Autodesk Inventor part; units mm, degrees
ref_plane "YZ Plane" through (0, 0, 0) normal (1, 0, 0) x (0, 1, 0)
ref_plane "XZ Plane" through (0, 0, 0) normal (0, 1, 0) x (-1, 0, 0)
ref_plane "XY Plane" through (0, 0, 0) normal (0, 0, 1) x (1, 0, 0)
sketch "Profile" plane through (0, 0, 0) normal (0, 0, 1) x (1, 0, 0)
  line L0 (-22.8, 0) -> (-22.8, 11)
  line L1 (-22.8, 11) -> (0, 11)
  line L2 (0, 11) -> (0.5774, 12)
  line L3 (0.5774, 12) -> (48.0774, 12)
  line L4 (48.0774, 12) -> (48.6547, 11)
  line L5 (48.6547, 11) -> (72.2, 11)
  line L6 (72.2, 11) -> (72.2, 0)
  line L7 (-22.8, 0) -> (0, 0)
  line L8 (0, 0) -> (0, 9)
  line L9 (0, 9) -> (64.2, 9)
  line L10 (64.2, 9) -> (64.2, 0)
  line L11 (64.2, 0) -> (72.2, 0)
  line L12 (-41.8, 0) -> (91.2, 0) construction
  line L13 (0, 11) -> (0, 9) construction
  dimension "BodyLength" = 95
  dimension "d1" = 11
  dimension "d3" = 120
  dimension "d4" = 120
  dimension "d5" = 47.5
  dimension "d6" = 22.8
  dimension "d16" = 8
  dimension "d29" = 1
  dimension "d30" = 9
revolve "ProfileRevolveFeature" add sketch "Profile" angle 360 about axis through (-10, 0, 0) along (1, 0, 0)
sketch "InsideHole" plane through (-22.8, 0, 0) normal (-1, 0, 0) x (0, 0, 1)
  circle A0 centre (0, 0) radius 9 construction
hole "InsideHoleFeature" at (-22.8, 0, 0) direction (1, 0, 0) diameter 19 end through all
chamfer "EndChamferFeature" distance 1 angle 45 1 edges at (-22.8, -11, 0)
sketch "CapMountHole" plane through (0, 0, 0) normal (0, 1, 0) x (-1, 0, 0)
  line L0 (-72.2, 11) -> (-72.2, -11) construction
  line L1 (15.2, 0) -> (-91.2, 0) construction
  circle A0 centre (-67.7, 0) radius 1.25
  point P0 (0, 0)
  dimension "d31" = 4.5
  dimension "d39" = 2.5
extrude "CapMountHoleFeature" cut sketch "CapMountHole" along normal through all both and the other way through all
equation "\"d5\" = 0.5 * BodyLength"
equation "\"d6\" = 0.24 * BodyLength"
properties part number "BackPair1PistonBody"
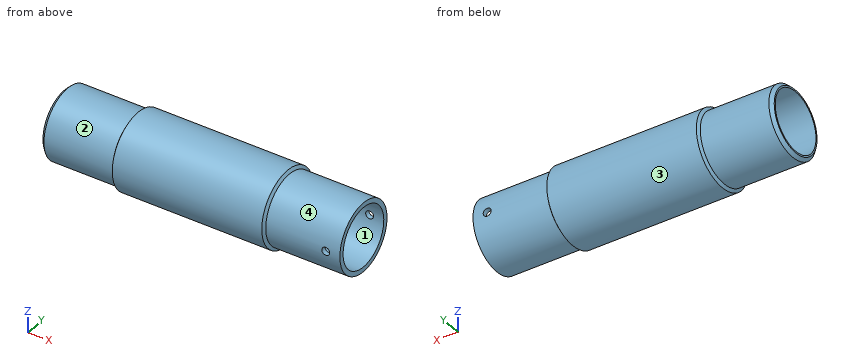
Could you check a few things on this model? Use its own coordinates, in mm. Face numbers are marked on the shaded views. A direction names the side the tool comes from. Round coordinates to 2 decimals unless told otherwise and drop trailing zeros. Order: outer loops, then holes, each group sorted by start corner. A loop starts at its lowest first (then second) coordinate and runs counter-clockwise, first axis right, second up.
(1) Imagine slicing it at B-B (z = 0). Write out the boundary of the cut face in (x, y), plus the area to 3 significant figures.
Response values:
outline: (-22.8, -10) - (-21.8, -11) - (0, -11) - (0.58, -12) - (48.08, -12) - (48.65, -11) - (66.45, -11) - (66.45, -9.5) - (-22.8, -9.5) - close; (-22.8, 9.5) - (66.45, 9.5) - (66.45, 11) - (48.65, 11) - (48.08, 12) - (0.58, 12) - (0, 11) - (-21.8, 11) - (-22.8, 10) - close; (68.95, -11) - (72.2, -11) - (72.2, -9.5) - (68.95, -9.5) - close; (68.95, 9.5) - (72.2, 9.5) - (72.2, 11) - (68.95, 11) - close
area: 373 mm2
(2) Imagine slicing it at A-A (y = 0). Write out the boundary of the cut face in (x, z), plus the area to 3 significant figures.
Response values:
outline: (-22.8, -10) - (-21.8, -11) - (0, -11) - (0.58, -12) - (48.08, -12) - (48.65, -11) - (72.2, -11) - (72.2, -9.5) - (-22.8, -9.5) - close; (-22.8, 9.5) - (72.2, 9.5) - (72.2, 11) - (48.65, 11) - (48.08, 12) - (0.58, 12) - (0, 11) - (-21.8, 11) - (-22.8, 10) - close
area: 380 mm2
(3) Imagine slicing it at D-D (x = 49.5). Write out the boundary of the cut face in (y, z).
Response values:
outline: circle Ø22 at (0, 0); hole circle Ø19 at (0, 0)
(4) If we mould it in two halves opening along Z, with no side actions, what happens to the marked faces 1 and 2? For each: released by +Z, released by -Z, zero draft, split by the parting line, or undercut.
Response values:
face 1: undercut
face 2: split by the parting line
(5) Which directions (+Z, -Z, +X, -X, +Y, -Y) give clear straight access to the entire face, cutting with the end or side of a thin tool? Please do the marked faces 3 and 4.
Response values:
face 3: +X, -X
face 4: +X
(6) Imagine slicing it at C-C (x = 67.7). Write out the boundary of the cut face in (y, z), plus the area to 3 significant figures.
Response values:
outline: (-10.93, -1.25) arc R11 ccw to (10.93, -1.25) - (9.42, -1.25) arc R9.5 cw to (-9.42, -1.25) - close; (-10.93, 1.25) - (-9.42, 1.25) arc R9.5 cw to (9.42, 1.25) - (10.93, 1.25) arc R11 ccw to start
area: 89.1 mm2
(7) Please list where these lines run through material, in increasing order: line 1 along X through (y, z) = (-9.75, 0); line 2 along Z through (x, y) = (4, 0); line 3 along Z through (x, y) = (-15, 2.5).
Response values:
line 1: x = -22.8 to 66.45, 68.95 to 72.2
line 2: z = -12 to -9.5, 9.5 to 12
line 3: z = -10.71 to -9.17, 9.17 to 10.71
(8) I'm going to push flat-ended pins straight in: pin 1 (10 mm diameter, centred on x = 32.5, y = 8, fed in from -Z); pin 2 (2 mm diameter, centred on x = 67.7, z = 0, fed in from +Y); pin 3 (2 mm diameter, centred on x = 56, y = 9, fed in from +Z); pin 4 (10 mm diameter, centred on x = 50.5, z = 5, fed in from +Y). Where does each tip first touch, or does it pass through?
Response values:
pin 1: stops at z = -11.62
pin 2: passes through
pin 3: stops at z = 7.55
pin 4: stops at y = 11.98
